Print and shaded views of the part. All mm, measured from the part's lowest x, y and z. Give positions to 0.01 mm unless a question says otherwise; leave off trailing zeros. Order: outer loops, then holes, each group sorted by start corner. A loop starts at its lowest first (then second) coordinate and runs counter-clockwise, first axis right, second up. Notation, with made-up numbers: (86, 88) - (123, 88) arc R7 ccw to (123, 92) - close; hole circle Ø6 at (-17, 89.5). An arc over 180 degrees is marked (long way). Answer in a Markdown table with one row per item.
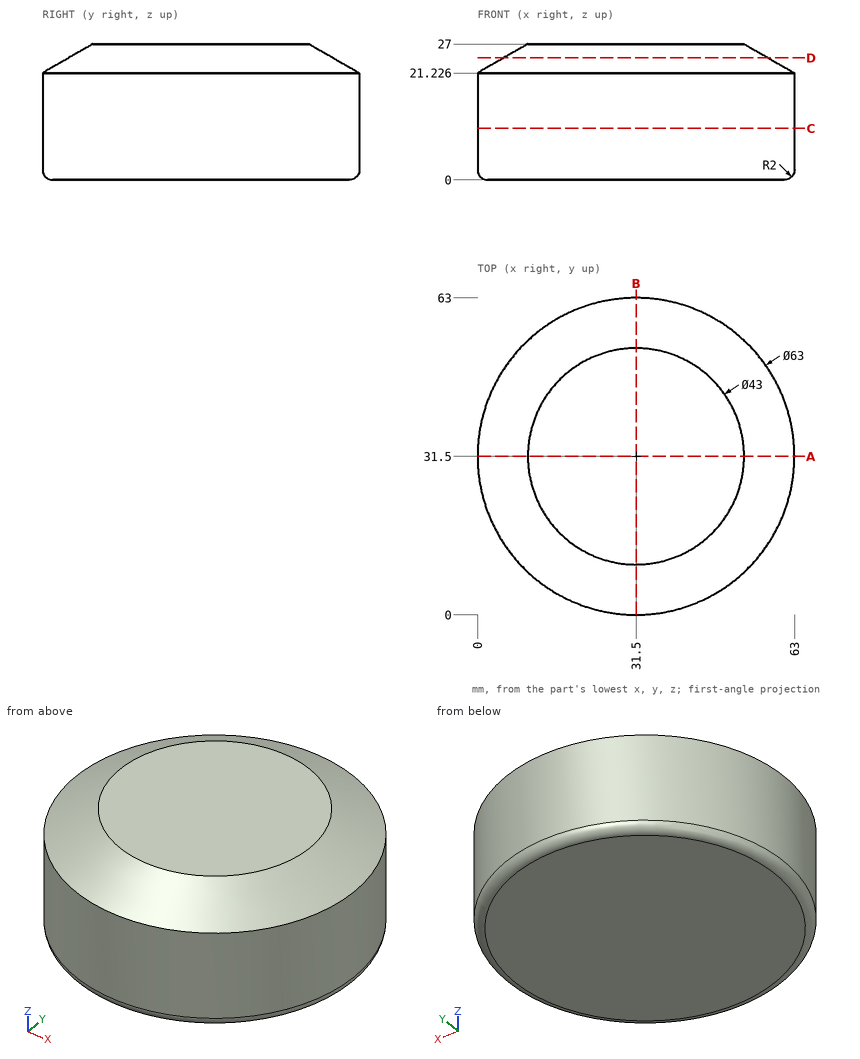
1. Probe line 1 (Z direction, x = 53, y = 31) (1 decimal); line 2 (X direction, y = 30.5, z = 6) (1 decimal); line 3 (Z direction, x = 28, y = 54.5). List the from-to ranges inside material, lowest first.
Check result:
| item | result |
|---|---|
| line 1 | z = 0 to 27 |
| line 2 | x = 0 to 63 |
| line 3 | z = 0 to 25.98 |
2. Cut at D-D on z = 24.25. Write the cut outline in (x, y).
Check result:
| item | result |
|---|---|
| outline | circle Ø52.53 at (31.5, 31.5) |
3. Cut at A-A on y = 31.5. Write the cut outline in (x, z), and give its area (3 significant figures).
Check result:
| item | result |
|---|---|
| outline | (0, 2) arc R2 ccw to (2, 0) - (61, 0) arc R2 ccw to (63, 2) - (63, 21.23) - (53, 27) - (10, 27) - (0, 21.23) - close |
| area | 1,640 mm² |
4. Cut at C-C on z = 10.25. Write the cut outline in (x, y).
Check result:
| item | result |
|---|---|
| outline | circle Ø63 at (31.5, 31.5) |
5. Drop flat-ended pins along their axis: P1, Ø6, axis at x = 36, z = 6, coming from the +Y side; P2, Ø6, axis at x = 22, z = 6, coming from the -Y side; P3, Ø4, axis at x = 54.5, z = 3.5, coming from the -Y side. Give the stop position or say it passes through.
Check result:
| item | result |
|---|---|
| P1 | stops at y = 62.96 |
| P2 | stops at y = 0.68 |
| P3 | stops at y = 8.02 |
